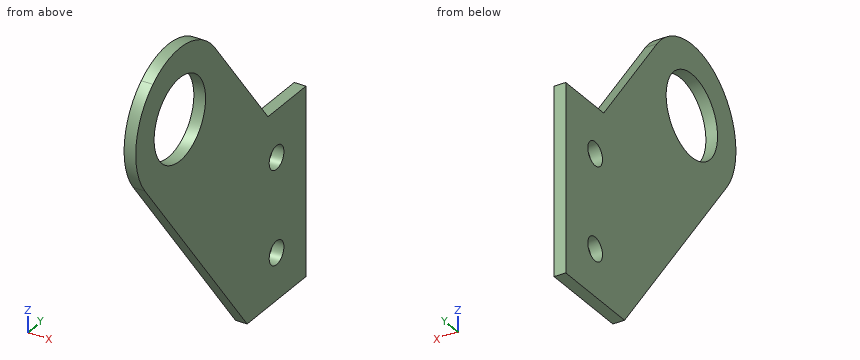
Autodesk Inventor part; units mm, degrees
ref_plane "YZ Plane" through (0, 0, 0) normal (1, 0, 0) x (0, 1, 0)
ref_plane "XZ Plane" through (0, 0, 0) normal (0, 1, 0) x (-1, 0, 0)
ref_plane "XY Plane" through (0, 0, 0) normal (0, 0, 1) x (1, 0, 0)
sketch "Sketch1" plane through (0, 0, 0) normal (1, 0, 0) x (0, 1, 0)
  line L0 (25.4, 50.8) -> (25.4, 0)
  line L1 (25.4, 0) -> (0, 0)
  line L2 (0, 0) -> (-55.7972, 72.5494)
  line L3 (25.4, 50.8) -> (8.9951, 50.8)
  line L4 (8.9951, 50.8) -> (-25.5962, 95.7768)
  line L5 (-25.5962, 95.7768) -> (-55.7972, 72.5494)
  circle A0 centre (-29.083, 69.0626) radius 11.1125
  line L6 (-40.6967, 84.1631) -> (-29.083, 69.0626) construction
  line L7 (25.4, 25.4) -> (-19.5349, 25.4) construction
  line L8 (12.7, 0) -> (12.7, 50.8) construction
  circle A1 centre (12.7, 12.7) radius 3.175
  circle A2 centre (12.7, 38.1) radius 3.175
  dimension "d9" = 38.1
  dimension "d10" = 19.05
  dimension "d11" = 50.8
  dimension "d12" = 29.083
  dimension "d13" = 43.6626
  dimension "d14" = 25.4
  dimension "d16" = 22.225
  dimension "d17" = 6.35
  dimension "d18" = 12.7
  dimension "d19" = 25.4
extrude "Extrusion1" add sketch "Sketch1" along normal blind 3.175
fillet "Fillet1" radius 19.05 2 edges at (1.5875, -25.5962, 95.7768) (1.5875, -55.7972, 72.5494)
properties part number "Rear roller plate"
CAD build for the part. Positions are in the model's coordinates, mm. Round coordinates to 2 decimals unless told otherwise and drop trailing zeros. Loops run counter-clockwise (first coordinate to the right, second up) from the corner with the lowest first, then second, coordinate; pieces in that order, holes last. Notation, with made-up numbers: (-32, 26) - (-16, 26) arc R35 ccw to (-16, 58) - close; hole circle Ø2 at (-35.5, 65.25). An arc over 180 degrees is marked (long way). Return JSON: item names as keys, results as strings. Group by question number.
Q1. Drill centre lines: line 1 along Z through (x, y) = (0.7, 12.7) (3 decimals); line 2 along Y through (x, z) = (1.15, 64); line 3 along Y through (x, z) = (2.6, 76). Where is each one in solid material? Low to high. Write a range as [from, to].
Q2. Band-saw the part on C-C on y = -22. Give the cut face in (x, z) (3 decimals), plus the area to 3 significant figures.
Q3. Flat gauge pins, fed straight in: pin 1 Ø1.5 at (x, y) = (2.5, -30.5) entering from -Z; pin 2 Ø7.5 at (y, z) = (12.7, 12.7) entering from -X; pin 3 Ø1.6 at (x, y) = (2.5, 18.5) entering from +Z. Where does each tip first touch, or does it go through?
Q4. Band-saw the part on B-B on z = 72. Give the cut face in (x, y) (3 decimals), plus the area to 3 significant figures.
Q5. Band-saw the part on D-D on x = 1.4. Give the number of separate pieces and of enclosed holes in the cut face, plus the area to 3 significant figures.
Q6. Band-saw the part on A-A on y = 12.7. Give the cut face in (x, z) (3 decimals).
Solutions:
{
 "1": {"line 1": "z = [0, 9.525], [15.875, 34.925], [41.275, 50.8]", "line 2": "y = [-47.45, -38.98], [-19.19, -1.16]", "line 3": "y = [-46.82, -37.76], [-20.4, -10.39]"},
 "2": {"outline": "(0, 28.605) - (3.175, 28.605) - (3.175, 60.5) - (0, 60.5) - close; (0, 77.625) - (3.175, 77.625) - (3.175, 86.747) - (0, 86.747) - close", "area": "130 mm^2"},
 "3": {"pin 1": "stops at z = 38.68", "pin 2": "stops at x = 0", "pin 3": "stops at z = 50.8"},
 "4": {"outline": "(0, -47.905) - (3.175, -47.905) - (3.175, -39.8) - (0, -39.8) - close; (0, -18.366) - (3.175, -18.366) - (3.175, -7.31) - (0, -7.31) - close", "area": "60.8 mm^2"},
 "5": {"separate pieces": "1", "enclosed holes": "3", "area": "3,280 mm^2"},
 "6": {"outline": "(0, 0) - (3.175, 0) - (3.175, 9.525) - (0, 9.525) - close; (0, 15.875) - (3.175, 15.875) - (3.175, 34.925) - (0, 34.925) - close; (0, 41.275) - (3.175, 41.275) - (3.175, 50.8) - (0, 50.8) - close"}
}
